from build123d import *

# Parameters (mm, degrees)
SKETCH1_W           = 95.40875
SKETCH1_H           = 69.85
BOSS_EXTRUDE1_DEPTH = 3.175
SKETCH1_4_R         = 3.96875
BOSS_EXTRUDE2_DEPTH = 15.875
SKETCH1_5_W         = 6.35
SKETCH1_5_H         = 12.7
BOSS_EXTRUDE3_DEPTH = 14.2875
SKETCH1_6_W         = 39.6875
SKETCH1_6_H         = 3.175
BOSS_EXTRUDE4_DEPTH = 11.1125
SKETCH1_8_R         = 1.5875
CUT_EXTRUDE4_DEPTH  = 104.830931221
SKETCH1_9_W         = 11.1125
SKETCH1_9_H         = 4.464487979
BOSS_EXTRUDE5_DEPTH = 11.1125
SKETCH1_10_W        = 9.525
SKETCH1_10_H        = 8.739789678
BOSS_EXTRUDE6_DEPTH = 12.7


with BuildPart() as part:
    # Sketch1 → Boss-Extrude1 (new body)
    with BuildSketch(Plane(origin=(0, 0, 0), x_dir=(1, 0, 0), z_dir=(0, 1, 0))):
        with Locations((-27.460937167, 34.925)):
            Rectangle(SKETCH1_W, SKETCH1_H)
    extrude(amount=BOSS_EXTRUDE1_DEPTH)

    # Sketch1<4> → Boss-Extrude2 (add)
    with BuildSketch(Plane(origin=(0, 0, 0), x_dir=(1, 0, 0), z_dir=(0, 1, 0))):
        with Locations(Location((-51.352812167, 14.2875, 0), (0, 0, 270))):
            Circle(SKETCH1_4_R)
        with Locations(Location((-4.486033595, 14.2875, 0), (0, 0, 270))):
            Circle(SKETCH1_4_R)
        with Locations(Location((9.130937833, 59.53125, 0), (0, 0, 270))):
            Circle(SKETCH1_4_R)
        with Locations(Location((-67.227812167, 59.53125, 0), (0, 0, 270))):
            Circle(SKETCH1_4_R)
    extrude(amount=BOSS_EXTRUDE2_DEPTH)

    # Sketch1<5> → Boss-Extrude3 (add)
    with BuildSketch(Plane(origin=(0, 0, 0), x_dir=(1, 0, 0), z_dir=(0, 1, 0))):
        with Locations((-70.402812167, 46.0375)):
            Rectangle(SKETCH1_5_W, SKETCH1_5_H)
        with Locations((-70.402812167, 22.225)):
            Rectangle(SKETCH1_5_W, SKETCH1_5_H)
        with Locations((15.480937833, 22.225)):
            Rectangle(SKETCH1_5_W, SKETCH1_5_H)
        with Locations((15.480937833, 46.0375)):
            Rectangle(SKETCH1_5_W, SKETCH1_5_H)
    extrude(amount=BOSS_EXTRUDE3_DEPTH)

    # Sketch1<6> → Boss-Extrude4 (add)
    with BuildSketch(Plane(origin=(0, 0, 0), x_dir=(1, 0, 0), z_dir=(0, 1, 0))):
        with Locations((-28.175312167, 65.0875)):
            Rectangle(SKETCH1_6_W, SKETCH1_6_H)
    extrude(amount=BOSS_EXTRUDE4_DEPTH)

    # Sketch1<8> → Cut-Extrude4 (cut, through all)
    with BuildSketch(Plane(origin=(0, 0, 0), x_dir=(1, 0, 0), z_dir=(0, 1, 0))):
        with Locations(Location((-71.990312167, 66.675, 0), (0, 0, 270))):
            Circle(SKETCH1_8_R)
        with Locations(Location((16.274687833, 3.175, 0), (0, 0, 90))):
            Circle(SKETCH1_8_R)
        with Locations(Location((16.274687833, 66.675, 0), (0, 0, 270))):
            Circle(SKETCH1_8_R)
        with Locations(Location((-71.990312167, 3.175, 0), (0, 0, 90))):
            Circle(SKETCH1_8_R)
    extrude(amount=CUT_EXTRUDE4_DEPTH, mode=Mode.SUBTRACT)

    # Sketch1<9> → Boss-Extrude5 (add)
    with BuildSketch(Plane(origin=(0, 0, 0), x_dir=(1, 0, 0), z_dir=(0, 1, 0))):
        with Locations((-36.271562167, 5.40724399)):
            Rectangle(SKETCH1_9_W, SKETCH1_9_H)
        with Locations((-21.984062167, 5.40724399)):
            Rectangle(SKETCH1_9_W, SKETCH1_9_H)
        with Locations((-7.696562167, 5.40724399)):
            Rectangle(SKETCH1_9_W, SKETCH1_9_H)
        with Locations((-50.559062167, 5.40724399)):
            Rectangle(SKETCH1_9_W, SKETCH1_9_H)
    extrude(amount=BOSS_EXTRUDE5_DEPTH)

    # Sketch1<10> → Boss-Extrude6 (add)
    with BuildSketch(Plane(origin=(0, 0, 0), x_dir=(1, 0, 0), z_dir=(0, 1, 0))):
        with Locations((-64.052812167, 5.957394839)):
            Rectangle(SKETCH1_10_W, SKETCH1_10_H)
        with Locations((5.955937833, 5.957394839)):
            Rectangle(SKETCH1_10_W, SKETCH1_10_H)
    extrude(amount=BOSS_EXTRUDE6_DEPTH)


solid = part.part
For this review, take the finished solid that the model builds, in its own axes (mm). A direction names the side the tool comes from. Give positions to 0.01 mm unless a question says otherwise; leave off trailing zeros. Loops run counter-clockwise (first coordinate to the right, second up) from the corner with the lowest first, then second, coordinate; pieces in that order, holes last.
Item 1: For line 1 along X through (y, z) = (11, -49); line 2 along Z through (x, y) = (-13, 5.25) (3 decimals); line 3 along X through (y, z) = (12.5, -6.5), list the stretches that pass through material, from the lowest coordinate up.
Item 2: Take a section at D-D, the plane x = -58. State the section outline as (y, z) points (3 decimals).
Item 3: Take a section at C-C, the plane y = 9. Give the number of separate pieces and of enclosed holes in the cut face, and give its area (3 significant figures).
Item 4: Draft analysis for pull direction X (two halves, no side actions). For faces 4 (the cylindrical face through (-50.161, 9.436, -10.502)), 5 (the flat face through (-64, 8, -10.327)), 6 (the flat face through (10.718, 8, -6)), state which applies: +X half, -X half, draft (parallel to the pull), parting line (faces both ways), or undercut.
Item 5: Take a section at B-B, the plane z = -24. State the section outline as (x, y) points (1 decimal).
Item 6: Insertion check: pin 1 (9 mm diameter, centred on y = 6, z = -21.5, fed in from -X); pin 2 (4 mm diameter, centred on x = -48.5, y = 7, fed in from +Z) (3 decimals); pin 3 (2.5 mm diameter, centred on y = 6.5, z = -7, fed in from +X); pin 4 (1 mm diameter, centred on x = -43, z = -47, fed in from +Y) (3 decimals). Each pin has a flat end and moves straight along its axis. Give the tip position at first contact, or say it passes through.
Item 7: Tool access review of faces 1 (the flat face through (6, 8, -1.588)), 2 (the flat face through (-13.253, 7, -5)), 3 (the flat face through (-28, 7, -63.5)): name each direction out of +Z, -Z, +X, -X, +Y, -Y from which nothing blocks a thin tool from reaching the whole face with its end or side.
Calculated:
1. line 1: x = -73.58 to -67.23, 12.31 to 18.66
1. line 2: z = -66.675 to -63.5, -7.639 to -3.175
1. line 3: x = -68.82 to -59.29, 1.19 to 10.72
2. outline: (0, -69.85) - (3.175, -69.85) - (3.175, 0) - (0, 0) - close
3. separate pieces: 15
3. enclosed holes: 0
3. area: 1,010 mm2
4. face 4: undercut
4. face 5: draft
4. face 6: +X half
5. outline: (-75.2, 0) - (20.2, 0) - (20.2, 3.2) - (18.7, 3.2) - (18.7, 14.3) - (12.3, 14.3) - (12.3, 3.2) - (-67.2, 3.2) - (-67.2, 14.3) - (-73.6, 14.3) - (-73.6, 3.2) - (-75.2, 3.2) - close
6. pin 1: stops at x = -75.17
6. pin 2: stops at z = -3.175
6. pin 3: stops at x = 10.72
6. pin 4: stops at y = 3.175
7. face 1: +Z, +X, -X, +Y
7. face 2: +Z, +Y
7. face 3: +Y
